Read the model definition and answer for the solid it produces. Units are mm, in the model's axes. A direction names the side the tool comes from. Round coordinates to 2 decimals unless told otherwise and drop trailing zeros. Order: outer loops, then holes, each group sorted by start corner. A loop starts at its lowest first (then second) coordinate and runs counter-clockwise, first axis right, second up. Notation, with made-up numbers: (-20, 81.5) -> (36, 81.5) arc R23 cw to (36, 119.5) -> close; hole circle Ø3 at (89, 2). An arc over 180 degrees is marked (long way). Answer as a JSON object with one key per item and string values. Group by question number.
Item 1: Consider probe 1 along Y at (x, z) = (281.5, 1384); probe 2 along Z at (x, y) = (1180, -191.5); probe 3 along Z at (x, y) = (934, -647). Determine where each line is inside the solid, lowest interval first. Write a range as from..to.
Item 2: Section C-C, the plane z = 167.64 is taken. Write down the section's boundary in (x, y), plus the area to 3 significant figures.
Item 3: For faces 5 (the flat face through (1042.289, -726, 50)), 6 (the flat face through (615, -434, 1610.36)), 7 (the flat face through (712.96, -115.23, 1645.42)), determine the directions among +Z, -Z, +X, -X, +Y, -Y from which every point of the face is accessible in a straight line to the end or side of a thin tool.
Item 4: Given P1, Ø19.5, axis at x = 326, y = -710, coming from the -Z side; P2, Ø21.5, axis at x = 921.5, z = 1657, coming from the +Y side, each flat-ended and moving along its own axis, determine where each tip first touches the part or whether it passes through.
Item 5: Section B-B, the plane y = -365 is taken. Write down the section's boundary in (x, z), plus the area to 3 significant figures.
Item 6: Section D-D, the plane z = 433 is taken. Write down the section's boundary in (x, y), plus the area to 3 significant figures.
Item 7: Section A-A, the plane x = 985 is taken. Write down the section's boundary in (y, z), plus the area to 3 significant figures.
Item 8: The mould has two halves that part along Z. Classify faces 1 (the flat face through (306, -326, 1681.48)), 2 (the flat face through (609, -726, 0)), 3 (the flat face through (396.24, -726, 50)), 4 (the flat face through (312, -27.94, 1645)): pulls with the +Z half, pulls with the -Z half, needs draft (parallel to the pull), parting line crosses it, or undercut.
from build123d import *

# Parameters (mm, degrees)
F0_W     = 1235.329
F0_H     = 1610.36
F0_W_2   = 203.2
F0_H_2   = 76.2
F1_DEPTH = 758.444
F2_W     = 628.904
F2_H     = 203.2
F3_DEPTH = 1235.33
F5_DEPTH = 71.12
F6_R     = 20.6375
F6_R_2   = 9.525
F7_DEPTH = 63.5


with BuildPart() as f1:
    # F0 (on Front) → F1 (new body)
    with BuildSketch(Plane.XZ):
        with Locations((617.6645, 805.18)):
            Rectangle(F0_W, F0_H)
        with Locations((294.64, 50.8)):
            Rectangle(F0_W_2, F0_H_2, mode=Mode.SUBTRACT)
        with Locations((940.689, 50.8)):
            Rectangle(F0_W_2, F0_H_2, mode=Mode.SUBTRACT)
    extrude(amount=F1_DEPTH)

    # F2 (on face) → F3 (cut, through all)
    with BuildSketch(Plane(origin=(0, 0, 0), x_dir=(0, -1, 0), z_dir=(-1, 0, 0))):
        with Locations((379.222, -5.842)):
            Rectangle(F2_W, F2_H)
    extrude(amount=-F3_DEPTH, mode=Mode.SUBTRACT)

    # F4 (on face) → F5 (join)
    with BuildSketch(Plane.XY.offset(1610.36)):
        Polygon((435.080191, -632.46), (612.14, -455.400191), (612.14, -204.999809), (435.080191, -27.94), (184.679809, -27.94), (7.62, -204.999809), (7.62, -455.400191), (184.679809, -632.46), align=None)
        Polygon((1050.649191, -632.46), (1227.709, -455.400191), (1227.709, -204.999809), (1050.649191, -27.94), (800.248809, -27.94), (623.189, -204.999809), (623.189, -455.400191), (800.248809, -632.46), align=None)
    extrude(amount=F5_DEPTH)

    # F6 (on face) → F7 (join)
    with BuildSketch(Plane.XZ.offset(758.444)):
        with Locations((1062.99, 167.64)):
            Circle(F6_R)
        with Locations((1062.99, 224.79)):
            Circle(F6_R_2)
    extrude(amount=F7_DEPTH)


solid = f1.part
Values found:
{
 "1": {"probe 1": "-758.44..0", "probe 2": "95.76..1681.48", "probe 3": "95.76..1610.36"},
 "2": {"outline": "(0, -758.44) -> (1042.35, -758.44) -> (1042.35, -821.94) -> (1083.63, -821.94) -> (1083.63, -758.44) -> (1235.33, -758.44) -> (1235.33, 0) -> (0, 0) -> close", "area": "940,000 mm2"},
 "3": {"face 5": "+Y, -Y", "face 6": "+Z", "face 7": "+Z, +Y"},
 "4": {"P1": "z = 0", "P2": "y = -27.94"},
 "5": {"outline": "(0, 95.76) -> (1235.33, 95.76) -> (1235.33, 1610.36) -> (1227.71, 1610.36) -> (1227.71, 1681.48) -> (623.19, 1681.48) -> (623.19, 1610.36) -> (612.14, 1610.36) -> (612.14, 1681.48) -> (7.62, 1681.48) -> (7.62, 1610.36) -> (0, 1610.36) -> close", "area": "1,960,000 mm2"},
 "6": {"outline": "(0, -758.44) -> (1235.33, -758.44) -> (1235.33, 0) -> (0, 0) -> close", "area": "937,000 mm2"},
 "7": {"outline": "(-758.44, 0) -> (-693.67, 0) -> (-693.67, 12.7) -> (-758.44, 12.7) -> close; (-758.44, 88.9) -> (-693.67, 88.9) -> (-693.67, 95.76) -> (-64.77, 95.76) -> (-64.77, 88.9) -> (0, 88.9) -> (0, 1610.36) -> (-27.94, 1610.36) -> (-27.94, 1681.48) -> (-632.46, 1681.48) -> (-632.46, 1610.36) -> (-758.44, 1610.36) -> close; (-64.77, 0) -> (0, 0) -> (0, 12.7) -> (-64.77, 12.7) -> close", "area": "1,190,000 mm2"},
 "8": {"face 1": "pulls with the +Z half", "face 2": "pulls with the -Z half", "face 3": "undercut", "face 4": "needs draft"}
}
